```python
from build123d import *

# Parameters (mm, degrees)
SKETCH009_W       = 13.18
SKETCH009_H       = 5.8
SKETCH009_W_2     = 12.5
SKETCH009_H_2     = 5.12
PAD005_DEPTH      = 2.66
PAD005_DEPTH_BACK = 11
SKETCH011_W       = 11.1
SKETCH011_H       = 1
SKETCH011_W_2     = 1
SKETCH011_H_2     = 3.6
PAD006_DEPTH      = 0.34
SKETCH012_W       = 11.5
SKETCH012_H       = 2
POCKET004_DEPTH   = 5
FILLET001_R       = 0.3


with BuildPart() as part:
    # Sketch009 → Pad005 (new body, two sides)
    with BuildSketch(Plane.XZ) as pad005_sk:
        with Locations((0, 4.64)):
            Rectangle(SKETCH009_W, SKETCH009_H)
        with Locations((0, 4.64)):
            Rectangle(SKETCH009_W_2, SKETCH009_H_2, mode=Mode.SUBTRACT)
    extrude(amount=PAD005_DEPTH)
    extrude(pad005_sk.sketch, amount=-PAD005_DEPTH_BACK)

    # Sketch011 → Pad006 (join)
    with BuildSketch(Plane.XZ.offset(2.66)):
        with Locations((0, 7.7)):
            Rectangle(SKETCH011_W, SKETCH011_H)
        with Locations((0, 1.58)):
            Rectangle(SKETCH011_W, SKETCH011_H)
        with Locations((-6.75, 4.64)):
            Rectangle(SKETCH011_W_2, SKETCH011_H_2)
        with Locations((6.75, 4.64)):
            Rectangle(SKETCH011_W_2, SKETCH011_H_2)
    extrude(amount=PAD006_DEPTH)

    # Sketch012 → Pocket004 (cut)
    with BuildSketch(Plane.XY):
        with Locations((0, 10)):
            Rectangle(SKETCH012_W, SKETCH012_H)
    extrude(amount=POCKET004_DEPTH, mode=Mode.SUBTRACT)

    # Fillet001
    fillet001_edges = [part.edges().sort_by_distance(p)[0] for p in [
        (-6.25, -3, 4.64),
        (0, -3, 7.2),
        (6.25, -3, 4.64),
        (0, -3, 2.08),
    ]]
    fillet(fillet001_edges, radius=FILLET001_R)


solid = part.part
```
Input: part model. Units: mm. Frame: model coordinates. A direction names the side the tool comes from. Coordinates: 2 decimals unless noted, no trailing zeros. Write each loop counter-clockwise with the first axis right and the second up, starting at its lowest first coordinate (ties: lowest second). Pieces come first, ordered by that corner, then holes.
1) Section C-C on y = 0. Output: boundary loops of the cut face in (x, z), and give its area (3 significant figures).
2) Pin query (flat end, axial travel): pin 1 Ø3 at (x, y) = (-2.5, 0.5) entering from -Z; pin 2 Ø3 at (x, y) = (-3.5, 1) entering from +Z; pin 3 Ø1.5 at (y, z) = (1, 5) entering from +X. Return the tip coordinate at first contact, or that it passes through.
3) Section B-B on x = 6. Output: boundary loops of the cut face in (y, z), and give its area (3 significant figures).
4) Section A-A on z = 7. Output: boundary loops of the cut face in (x, y).
5) Material intervals for line 1 along Z through (x, y) = (3.5, 3); line 2 along X through (y, z) = (-1, 3); line 3 along Y through (x, z) = (2, 1.5), sorted ascending.
6) Mould query, pull axis Z, two halves, no side actions, for faces 1 (the flat face through (6.25, 4, 5)), 2 (the flat face through (0, 4, 1.74)), 3 (the flat face through (0, 4, 2.08)), 4 (the flat face through (6.59, 4, 5)). Classes: pulls with the +Z half, pulls with the -Z half, needs draft (parallel to the pull), parting line crosses it, or undercut.
7) Set-up query: faces 5 (the flat face through (0, 4, 7.2)), 6 (the flat face through (6.4, -2.66, 7.1)), 7 (the flat face through (-6.4, -2.66, 7.1)). Return all of +Z, -Z, +X, -X, +Y, -Y with unobstructed straight access to the full face (end or side cutting, diameter ignored); none if empty.
8) Section D-D on y = 10. Output: boundary loops of the cut face in (x, z).
Check result:
1. outline: (-6.59, 1.74) - (6.59, 1.74) - (6.59, 7.54) - (-6.59, 7.54) - close; hole (-6.25, 2.08) - (6.25, 2.08) - (6.25, 7.2) - (-6.25, 7.2) - close
1. area: 12.4 mm2
2. pin 1: stops at z = 1.74
2. pin 2: stops at z = 7.54
2. pin 3: stops at x = 6.59
3. outline: (-2.66, 1.74) - (11, 1.74) - (11, 2.08) - (-2.66, 2.08) - close; (-2.66, 7.2) - (11, 7.2) - (11, 7.54) - (-2.66, 7.54) - close
3. area: 9.29 mm2
4. outline: (-6.59, -2.66) - (-6.25, -2.66) - (-6.25, 11) - (-6.59, 11) - close; (6.25, -2.66) - (6.59, -2.66) - (6.59, 11) - (6.25, 11) - close
5. line 1: z = 1.74 to 2.08, 7.2 to 7.54
5. line 2: x = -6.59 to -6.25, 6.25 to 6.59
5. line 3: y = -3 to -2.66
6. face 1: undercut
6. face 2: pulls with the -Z half
6. face 3: undercut
6. face 4: needs draft
7. face 5: +Y, -Y
7. face 6: +Z, +X, -Y
7. face 7: +Z, -X, -Y
8. outline: (-6.59, 1.74) - (-5.75, 1.74) - (-5.75, 2.08) - (-6.25, 2.08) - (-6.25, 7.2) - (6.25, 7.2) - (6.25, 2.08) - (5.75, 2.08) - (5.75, 1.74) - (6.59, 1.74) - (6.59, 7.54) - (-6.59, 7.54) - close
